Could you check a few things on this model? Use its own coordinates, in mm. Round coordinates to 2 decimals unless told otherwise and drop trailing zeros. Write each loop counter-clockwise with the first axis right and the second up, starting at its lowest first coordinate (ties: lowest second). Pieces come first, ordered by that corner, then holes. Notation, with made-up numbers: (-22.75, 50) -> (5.25, 50) arc R9 cw to (5.25, 55) -> close; hole circle Ø9 at (78.5, 72.5). An arc over 180 degrees is marked (long way). Answer as CSV lines item,"result". Start each with the question number.
Q1. Will these pins go through, and if not, where does the flat tip stop? pin 1 Ø1.2 at (x, y) = (63, 2) entering from -Z; pin 2 Ø2 at (x, y) = (68.5, 1) entering from +Z; pin 3 Ø1.2 at (y, z) = (3, -3) entering from -X.
Q2. Imagine slicing it at B-B on z = 8. Please give me the cut outline in (x, y), and give its area (3 significant figures).
Q3. If I drill on line 1 (Z direction, x = 66.5, y = 2.05); line 2 (X direction, y = 1.8, z = -2); line 3 (X direction, y = 2.2, z = 6.75), over which ranges is the centre line in solid material (lowest first)? Write a range as [from, to].
Q4. Imagine slicing it at C-C on x = 1.5. Please give me the cut outline in (y, z).
from build123d import *

# Parameters (mm, degrees)
SKETCH1_W           = 66
SKETCH1_H           = 25
BOSS_EXTRUDE1_DEPTH = 4
SKETCH2_W           = 4
SKETCH2_H           = 5
BOSS_EXTRUDE2_DEPTH = 4
LPATTERN1_COUNT     = 2
LPATTERN1_PITCH     = 10
SKETCH3_W           = 10
SKETCH3_H           = 4
BOSS_EXTRUDE3_DEPTH = 4
LPATTERN2_COUNT     = 2
LPATTERN2_PITCH     = 20
LPATTERN2_COL_COUNT = 2
LPATTERN2_COL_PITCH = 20
SKETCH5_W           = 4
SKETCH5_H           = 6
SKETCH5_H_2         = 4
BOSS_EXTRUDE4_DEPTH = 4


with BuildPart() as part:
    # Sketch1 → Boss-Extrude1 (new body)
    with BuildSketch(Plane(origin=(0, 0, 0), x_dir=(1, 0, 0), z_dir=(0, 1, 0))):
        with Locations((33, -12.5)):
            Rectangle(SKETCH1_W, SKETCH1_H)
    extrude(amount=BOSS_EXTRUDE1_DEPTH)

    # Sketch2 → Boss-Extrude2 (add, through all)
    with BuildSketch(Plane(origin=(0, 4, 0), x_dir=(1, 0, 0), z_dir=(0, 1, 0))):
        with Locations((-2, -7.5)):
            Rectangle(SKETCH2_W, SKETCH2_H)
    boss_extrude2 = extrude(amount=-BOSS_EXTRUDE2_DEPTH)

    # LPattern1: Boss-Extrude2 ×2
    with Locations(*[(0, 0, i * LPATTERN1_PITCH) for i in range(1, LPATTERN1_COUNT)]):
        add(boss_extrude2)

    # Sketch3 → Boss-Extrude3 (add, through all)
    with BuildSketch(Plane(origin=(0, 4, 0), x_dir=(1, 0, 0), z_dir=(0, 1, 0))):
        with Locations((33, 2)):
            Rectangle(SKETCH3_W, SKETCH3_H)
    boss_extrude3 = extrude(amount=-BOSS_EXTRUDE3_DEPTH)

    # LPattern2: Boss-Extrude3 ×2
    with Locations(*[(i * LPATTERN2_PITCH, 0, 0) for i in range(1, LPATTERN2_COUNT)]):
        add(boss_extrude3)

    # LPattern2 col: Boss-Extrude3 ×2
    with Locations(*[(-i * LPATTERN2_COL_PITCH, 0, 0) for i in range(1, LPATTERN2_COL_COUNT)]):
        add(boss_extrude3)

    # Sketch5 → Boss-Extrude4 (add, through all)
    with BuildSketch(Plane(origin=(0, 4, 0), x_dir=(1, 0, 0), z_dir=(0, 1, 0))):
        with Locations((68, -3)):
            Rectangle(SKETCH5_W, SKETCH5_H)
        with Locations((68, -12)):
            Rectangle(SKETCH5_W, SKETCH5_H_2)
        with Locations((68, -20)):
            Rectangle(SKETCH5_W, SKETCH5_H_2)
    extrude(amount=-BOSS_EXTRUDE4_DEPTH)


solid = part.part
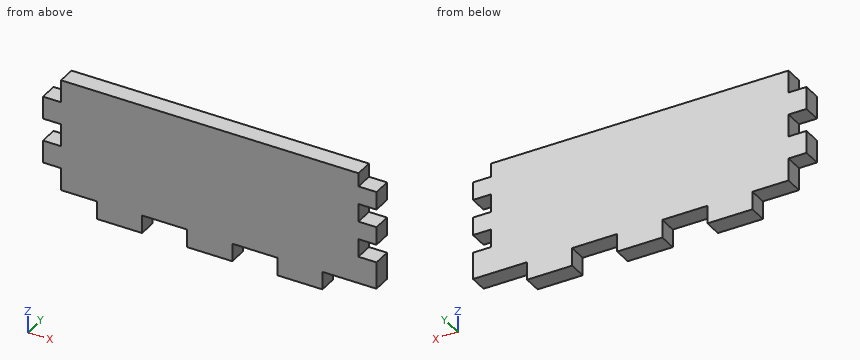
Checks:
1,pin 1,"z = 0"
1,pin 2,"z = 22"
1,pin 3,"x = 8"
2,outline,"(-4, 0) -> (66, 0) -> (66, 4) -> (-4, 4) -> close"
2,area,"280 mm^2"
3,line 1,"[0, 6], [10, 14], [18, 22]"
3,line 2,"[8, 18], [28, 38], [48, 58]"
3,line 3,"[-4, 66]"
4,outline,"(0, 0) -> (4, 0) -> (4, 25) -> (0, 25) -> close"
